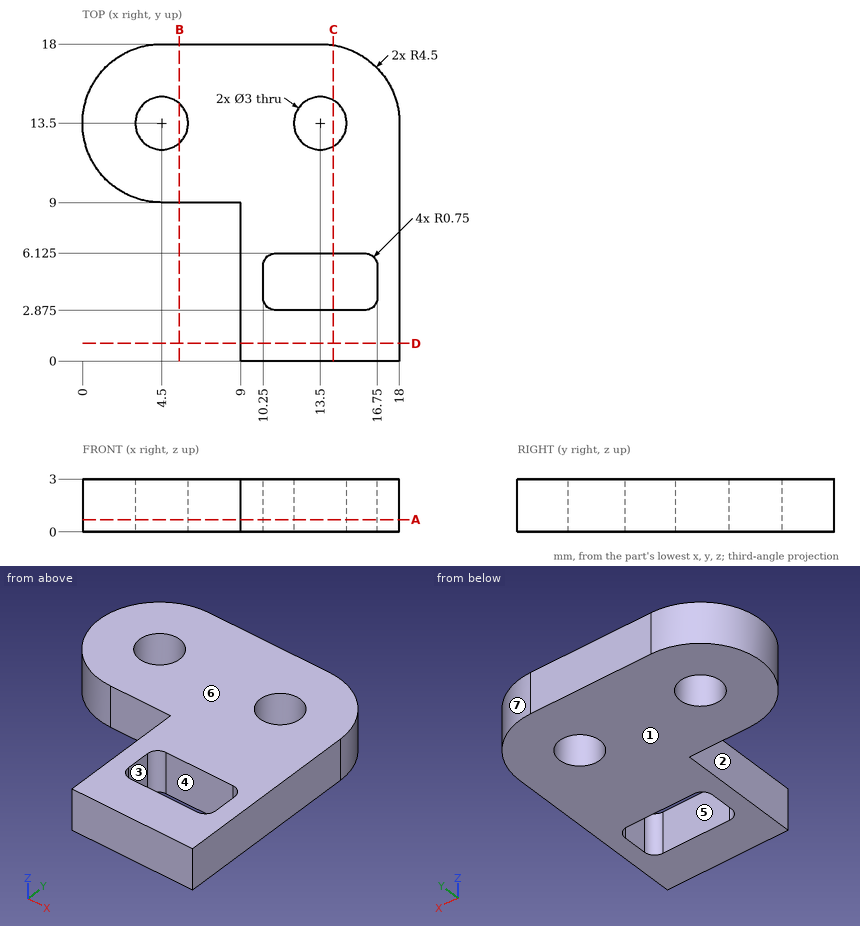
Answer from the drawing. Dimensions are ordinates in mm from the lowest x, y and z of the part. A direction names the side the tool comes from. Round coordinates to 2 decimals unless told otherwise and drop trailing zeros. Order: outer loops, then holes, each group sorted by start corner. A loop starts at its lowest first (then second) coordinate and runs counter-clockwise, first axis right, second up. Notation, with made-up numbers: (-14.75, -0.75) - (38.25, -0.75) arc R28 cw to (38.25, 34.25) - close; hole circle Ø9 at (50, 38.25). An arc over 180 degrees is marked (long way). Put each result on its own line as item: value. Start each with the question number.
(1) Find section C-C (x = 14.25). Give the vertices of the cut face in (y, z) (3 decimals), plus the area to 3 significant figures.
(2) Straight lines are drawn through the part: probe 1 along X at (y, z) = (13.5, 1.65); probe 2 along X at (y, z) = (4.5, 0.55); probe 3 along X at (y, z) = (12.5, 2.65). For each, find the intervals that lie inside material, in ascending order. Write a range as from..to.
(3) Determine the mould class of the marked faces 4, 5, 6 and 7 for opening direction X: released by +X, released by -X, zero draft, split by the parting line, or undercut.
(4) For the marked faces 1, 2 and 3, determine the directions among +Z, -Z, +X, -X, +Y, -Y from which every point of the face is accessible in a straight line to the end or side of a thin tool.
(5) Find section D-D (y = 1). Give the vertices of the cut face in (x, z), plus the area to 3 significant figures.
(6) Find section B-B (x = 5.5). Give the vertices of the cut face in (y, z).
(7) Given P1, Ø0.9, axis at y = 3.5, z = 2, coming from the -X side, flat-ended and moving along its own axis, determine where the tip first touches the part or whether it passes through.
(8) Find section A-A (z = 0.7). Give the vertices of the cut face in (x, y) (3 decimals).
Reply:
1. outline: (0, 0) - (2.875, 0) - (2.875, 3) - (0, 3) - close; (6.125, 0) - (12.201, 0) - (12.201, 3) - (6.125, 3) - close; (14.799, 0) - (17.937, 0) - (17.937, 3) - (14.799, 3) - close
1. area: 36.3 mm^2
2. probe 1: 0..3, 6..12, 15..18
2. probe 2: 9..10.25, 16.75..18
2. probe 3: 0.11..3.38, 5.62..12.38, 14.62..18
3. face 4: undercut
3. face 5: undercut
3. face 6: zero draft
3. face 7: released by +X
4. face 1: -Z, +X, -X, +Y, -Y
4. face 2: +Z, -Z, -X, -Y
4. face 3: +Z, -Z
5. outline: (9, 0) - (18, 0) - (18, 3) - (9, 3) - close
5. area: 27.0 mm^2
6. outline: (9, 0) - (12.38, 0) - (12.38, 3) - (9, 3) - close; (14.62, 0) - (18, 0) - (18, 3) - (14.62, 3) - close
7. P1: x = 9
8. outline: (4.5, 9) - (9, 9) - (9, 0) - (18, 0) - (18, 13.5) arc R4.5 ccw to (13.5, 18) - (4.5, 18) arc R4.5 ccw to start; hole circle Ø3 at (4.5, 13.5); hole (10.25, 3.625) arc R0.75 ccw to (11, 2.875) - (16, 2.875) arc R0.75 ccw to (16.75, 3.625) - (16.75, 5.375) arc R0.75 ccw to (16, 6.125) - (11, 6.125) arc R0.75 ccw to (10.25, 5.375) - close; hole circle Ø3 at (13.5, 13.5)
